Could you check a few things on this drawing? It's one solid part, dimensions in mm from its lowest x, y, z. A direction names the side the tool comes from. Give positions to 0.01 mm unless a question says otherwise; leave off trailing zeros. Order: outer loops, then holes, each group sorted by start corner. A loop starts at its lowest first (then second) coordinate and runs counter-clockwise, first axis right, second up.
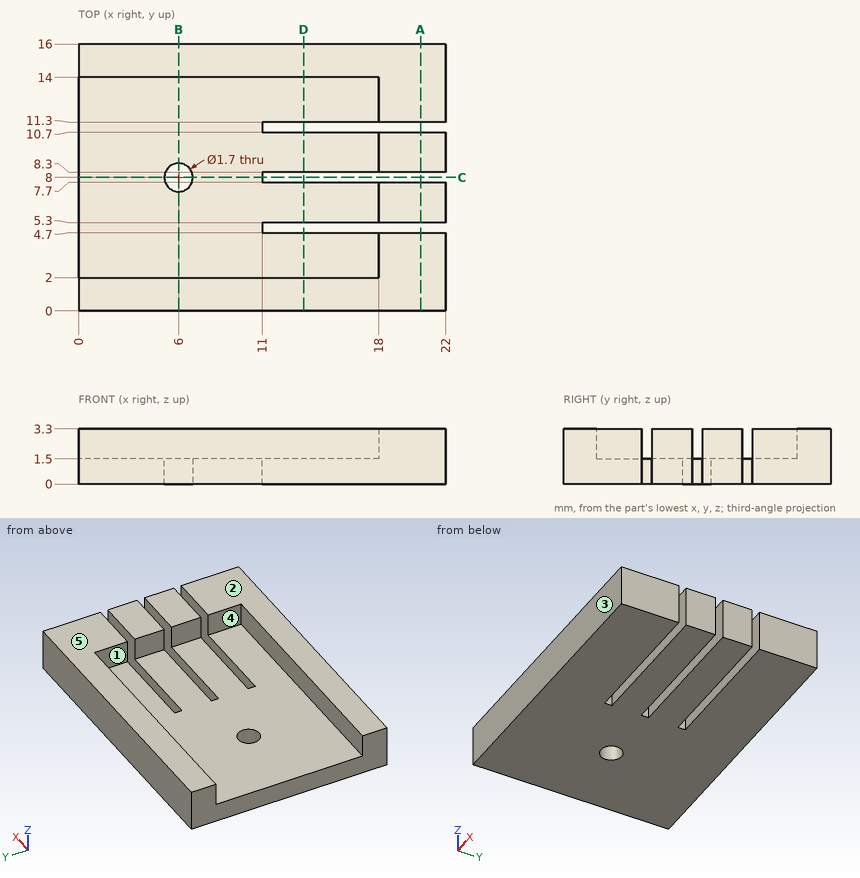
1) I'm going to push flat-ended pins straight in: pin 1 Ø1.5 at (x, y) = (6, 7) entering from +Z; pin 2 Ø0.5 at (y, z) = (12.5, 2.5) entering from -X; pin 3 Ø0.5 at (y, z) = (11, 1) entering from +X. Where does each tip first touch, or does it pass through?
2) Suppose I cut it at B-B (x = 6). Please give me the cut outline in (y, z), and give its area (4 significant figures).
3) Which directions (+Z, -Z, +X, -X, +Y, -Y) give clear straight access to the entire face, cutting with the end or side of a thin tool? Please do the marked faces 4 and 5.
4) We'd pull the mould along Y, two halves only. Please class the marked faces 1, 2 and 3: +Y half, -Y half, draft (parallel to the pull), parting line (faces both ways), or undercut.
5) Suppose I cut it at C-C (y = 8). Please give me the cut outline in (x, z), and give its area (4 significant figures).
6) Suppose I cut it at D-D (x = 13.5). Please give me the cut outline in (y, z), and give its area (3 significant figures).
7) If I drill on line 1 (Y direction, x = 14, z = 0.3); line 2 (Y direction, x = 13, z = 2); line 3 (Y direction, x = 6, z = 0.9), over which ranges is the centre line in solid material (lowest first)?
8) Suppose I cut it at A-A (x = 20.5). Please give me the cut outline in (y, z).
Results:
1. pin 1: stops at z = 1.5
1. pin 2: stops at x = 18
1. pin 3: stops at x = 11
2. outline: (0, 0) - (7.15, 0) - (7.15, 1.5) - (2, 1.5) - (2, 3.3) - (0, 3.3) - close; (8.85, 0) - (16, 0) - (16, 3.3) - (14, 3.3) - (14, 1.5) - (8.85, 1.5) - close
2. area: 28.65 mm2
3. face 4: +Z, -X
3. face 5: +Z, +X, -X, +Y, -Y
4. face 1: undercut
4. face 2: draft
4. face 3: -Y half
5. outline: (0, 0) - (5.15, 0) - (5.15, 1.5) - (0, 1.5) - close; (6.85, 0) - (11, 0) - (11, 1.5) - (6.85, 1.5) - close
5. area: 13.95 mm2
6. outline: (0, 0) - (4.7, 0) - (4.7, 1.5) - (2, 1.5) - (2, 3.3) - (0, 3.3) - close; (5.3, 0) - (7.7, 0) - (7.7, 1.5) - (5.3, 1.5) - close; (8.3, 0) - (10.7, 0) - (10.7, 1.5) - (8.3, 1.5) - close; (11.3, 0) - (16, 0) - (16, 3.3) - (14, 3.3) - (14, 1.5) - (11.3, 1.5) - close
6. area: 28.5 mm2
7. line 1: y = 0 to 4.7, 5.3 to 7.7, 8.3 to 10.7, 11.3 to 16
7. line 2: y = 0 to 2, 14 to 16
7. line 3: y = 0 to 7.15, 8.85 to 16
8. outline: (0, 0) - (4.7, 0) - (4.7, 3.3) - (0, 3.3) - close; (5.3, 0) - (7.7, 0) - (7.7, 3.3) - (5.3, 3.3) - close; (8.3, 0) - (10.7, 0) - (10.7, 3.3) - (8.3, 3.3) - close; (11.3, 0) - (16, 0) - (16, 3.3) - (11.3, 3.3) - close
